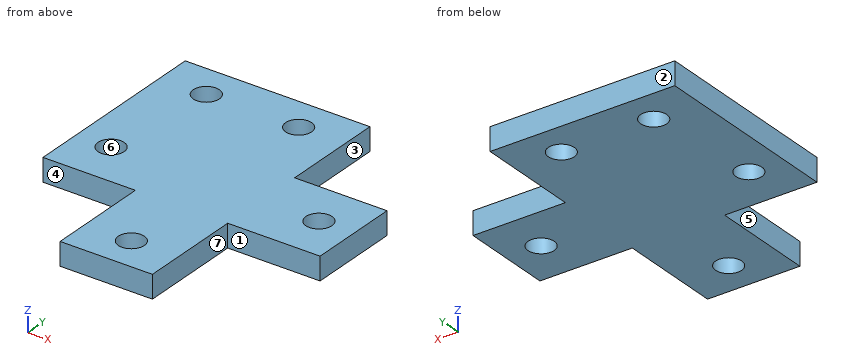
from build123d import *

# Parameters (mm, degrees)
SKETCH3_R             = 1
BOSS_EXTRUDE1_DEPTH   = 2
F_4_40_TAPPED_HOLE1_D = 2.2606


with BuildPart() as part:
    # Sketch3 → Boss-Extrude1 (new body)
    with BuildSketch(Plane.XY):
        Polygon((8, 0), (-8, 0), (-8, -17), (0, -17), (0, -26), (8, -26), (8, -17), (16, -17), (16, -9), (8, -9), align=None)
        with Locations((4, -3)):
            Circle(SKETCH3_R, mode=Mode.SUBTRACT)
        with Locations((-4, -3)):
            Circle(SKETCH3_R, mode=Mode.SUBTRACT)
        with Locations((-5, -13)):
            Circle(SKETCH3_R, mode=Mode.SUBTRACT)
        with Locations((13, -13)):
            Circle(SKETCH3_R, mode=Mode.SUBTRACT)
        with Locations((4, -23)):
            Circle(SKETCH3_R, mode=Mode.SUBTRACT)
    extrude(amount=BOSS_EXTRUDE1_DEPTH)

    # #4-40 Tapped Hole1 (through all)
    with Locations(Plane(origin=(-5, -13, 2), x_dir=(1, 0, 0), z_dir=(0, 0, 1))):
        with Locations((0, 0), (18, 0), (9, -10), (9, 10), (1, 10)):
            Hole(F_4_40_TAPPED_HOLE1_D / 2)


solid = part.part
Design review of the part built by this model. Coordinates are the model's own, in mm. Face numbers are marked on the shaded views. A direction names the side the tool comes from. Round coordinates to 2 decimals unless told otherwise and drop trailing zeros. Loops run counter-clockwise (first coordinate to the right, second up) from the corner with the lowest first, then second, coordinate; pieces in that order, holes last. Notation, with made-up numbers: M 83,57.5 L 110,57.5 A30 ccw 110,95.5 Z; hole C 32,34.25 d1. An arc over 180 degrees is marked long. Answer as a JSON object with one key per item and string values.
Item 1: Wall thickness on L1, parallel to Y at x = 4, z = 1.05; L2, parallel to Y at x = -4, z = 0.9; L3, parallel to X at y = -13.25, z = 1.6: over which ranges is each line inside the solid? List them lowest first. Write a range as from..to.
Answer sheet:
{"L1": "y = -26..-24.13, -21.87..-4.13, -1.87..0", "L2": "y = -17..-13.53, -12.47..-4.13, -1.87..0", "L3": "x = -8..-6.1, -3.9..11.9, 14.1..16"}
Item 2: The part is to be moulded in two halves that separate along X. For the marked faces 4, 5, 6 and 7, say which applies: pulls with the +X half, pulls with the -X half, needs draft (parallel to the pull), parting line crosses it, or undercut.
Answer sheet:
{"face 4": "needs draft", "face 5": "pulls with the -X half", "face 6": "undercut", "face 7": "pulls with the +X half"}
Item 3: We need section C-C on y = -13.75. Give the boundary of the cut face in (x, z), and give its area (3 significant figures).
Answer sheet:
{"outline": "M -8,0 L -5.85,0 L -5.85,2 L -8,2 Z; M -4.15,0 L 12.15,0 L 12.15,2 L -4.15,2 Z; M 13.85,0 L 16,0 L 16,2 L 13.85,2 Z", "area": "41.2 mm^2"}
Item 4: Machinability: for the marked faces 1, 2 and 3, which of the approach directions +Z, -Z, +X, -X, +Y, -Y give a long, thin tool a straight path to every point of the face, cutting with its end or side? Answer none if there is none.
Answer sheet:
{"face 1": "+Z, -Z, +X, -Y", "face 2": "+Z, -Z, +X, -X, +Y", "face 3": "+Z, -Z, +X, +Y"}
Item 5: We need section B-B on z = 1.55. Give the boundary of the cut face in (x, y), and give its area (3 significant figures).
Answer sheet:
{"outline": "M -8,-17 L 0,-17 L 0,-26 L 8,-26 L 8,-17 L 16,-17 L 16,-9 L 8,-9 L 8,0 L -8,0 Z; hole C -5,-13 d2.26; hole C -4,-3 d2.26; hole C 4,-23 d2.26; hole C 4,-3 d2.26; hole C 13,-13 d2.26", "area": "388 mm^2"}
Item 6: Clearance check with flat-ended pins moving along their axes: P1, Ø1, axis at y = -20, z = 1.5, coming from the +X side; P2, Ø1, axis at x = 13, z = 1, coming from the +Y side. State where each tip first meets the part, or that it passes through.
Answer sheet:
{"P1": "stops at x = 8", "P2": "stops at y = -9"}
Item 7: We need section D-D on y = -18. Give the boundary of the cut face in (x, z), and give its area (3 significant figures).
Answer sheet:
{"outline": "M 0,0 L 8,0 L 8,2 L 0,2 Z", "area": "16.0 mm^2"}
Item 8: We need section A-A on x = 4. Give the boundary of the cut face in (y, z).
Answer sheet:
{"outline": "M -26,0 L -24.13,0 L -24.13,2 L -26,2 Z; M -21.87,0 L -4.13,0 L -4.13,2 L -21.87,2 Z; M -1.87,0 L 0,0 L 0,2 L -1.87,2 Z"}
